Could you check a few things on this model? Use its own coordinates, in mm. A direction names the side the tool comes from. Round coordinates to 2 decimals unless told otherwise and drop trailing zeros. Loops run counter-clockwise (first coordinate to the right, second up) from the corner with the lowest first, then second, coordinate; pieces in that order, holes last. Notation, with made-up numbers: (59, 84) -> (66, 84) arc R18 cw to (66, 96) -> close; hole circle Ø11 at (-13, -22.5). An arc over 180 degrees is marked (long way). One line per item, written item: value.
```python
from build123d import *

# Parameters (mm, degrees)
F0_W      = 25
F0_H      = 90
F1_DEPTH  = 2
F2_R      = 2
F3_DEPTH  = 25
F4_W      = 25
F4_H      = 5
F5_DEPTH  = 2
F6_W      = 25
F6_H      = 2
F7_DEPTH  = 63
F8_R      = 5
F10_DEPTH = 25


with BuildPart() as f1:
    # F0 (on Front) → F1 (new body)
    with BuildSketch(Plane.XZ):
        Rectangle(F0_W, F0_H)
    extrude(amount=F1_DEPTH)

    # F2 (on face) → F3 (cut)
    with BuildSketch(Plane.XZ.offset(2)):
        with Locations((7.5, 25)):
            Circle(F2_R)
        with Locations((-6.5, -3)):
            Circle(F2_R)
    extrude(amount=-F3_DEPTH, mode=Mode.SUBTRACT)

    # F4 (on face) → F5 (join)
    with BuildSketch(Plane.XZ.offset(2)):
        with Locations((0, 47.5)):
            Rectangle(F4_W, F4_H)
    extrude(amount=-F5_DEPTH)

    # F6 (on face) → F7 (join)
    with BuildSketch(Plane.XZ.offset(2)):
        with Locations((0, 49)):
            Rectangle(F6_W, F6_H)
    extrude(amount=F7_DEPTH)

    # F8
    f8_edges = [f1.edges().sort_by_distance(p)[0] for p in [
        (-12.5, -65, 49),
        (12.5, -65, 49),
    ]]
    fillet(f8_edges, radius=F8_R)

    # F9 (on face) → F10 (cut)
    with BuildSketch(Plane.XY.offset(50)):
        with BuildLine():
            Line((-7.5, -49.8), (7.5, -49.8))
            ThreePointArc((7.5, -49.8), (10.5, -46.8), (7.5, -43.8))
            Line((7.5, -43.8), (-7.5, -43.8))
            ThreePointArc((-7.5, -43.8), (-10.5, -46.8), (-7.5, -49.8))
        make_face()
    extrude(amount=-F10_DEPTH, mode=Mode.SUBTRACT)


solid = f1.part
```
(1) We'd pull the mould along X, two halves only. Please class faces 1 (the face through (-11.07, -63.5, 49.01)), 2 (the face through (10.5, -46.9, 49)), 3 (the face through (0, 0, 3)): +X half, -X half, draft (parallel to the pull), parting line (faces both ways), or undercut.
Results below:
face 1: -X half
face 2: undercut
face 3: draft
(2) For pin 1 Ø2 at (x, y) = (-9.5, -9.5) entering from -Z; pin 2 Ø12.5 at (x, z) = (-4, 6.5) entering from -Y, each with a flat end and sliding along its axis, tell me the tip position at first contact or that it passes through.
Results below:
pin 1: stops at z = 48
pin 2: stops at y = -2
(3) Please list where these lines run through material, in increasing order: L1, parallel to Z at x = 8.5, y = -12; L2, parallel to Y at x = -1.5, z = -20; L3, parallel to Z at x = -6.5, y = -1.45.
Results below:
L1: z = 48 to 50
L2: y = -2 to 0
L3: z = -45 to -5, -1 to 50
(4) Imagine slicing it at C-C on x = -5.5. Write out the boundary of the cut face in (y, z).
Results below:
outline: (-65, 48) -> (-49.8, 48) -> (-49.8, 50) -> (-65, 50) -> close; (-43.8, 48) -> (-2, 48) -> (-2, -1.27) -> (0, -1.27) -> (0, 50) -> (-43.8, 50) -> close; (-2, -45) -> (0, -45) -> (0, -4.73) -> (-2, -4.73) -> close
(5) On a 3-axis mill with a long thin cutter (end or side, diameter ignored), from which of +Z, -Z, +X, -X, +Y, -Y can I reach the whole of each face in a straight line? I mean faces 4 (the face through (0, -2, 2)), 5 (the face through (-12.5, -1, 23)), 6 (the face through (0, -49.8, 49)). Say none if no direction works.
Results below:
face 4: -Z, +X, -X, -Y
face 5: +Z, -Z, -X, +Y, -Y
face 6: +Z, -Z
(6) Imagine slicing it at B-B on z = -3. Write out the boundary of the cut face in (x, y).
Results below:
outline: (-12.5, -2) -> (-8.5, -2) -> (-8.5, 0) -> (-12.5, 0) -> close; (-4.5, -2) -> (12.5, -2) -> (12.5, 0) -> (-4.5, 0) -> close
(7) Imagine slicing it at D-D on y = -8.5. Write out the boundary of the cut face in (x, z).
Results below:
outline: (-12.5, 48) -> (12.5, 48) -> (12.5, 50) -> (-12.5, 50) -> close
(8) Imagine slicing it at A-A on x = 1. Write out the boundary of the cut face in (y, z), then the cut area to 3 significant figures.
Results below:
outline: (-65, 48) -> (-49.8, 48) -> (-49.8, 50) -> (-65, 50) -> close; (-43.8, 48) -> (-2, 48) -> (-2, -45) -> (0, -45) -> (0, 50) -> (-43.8, 50) -> close
area: 304 mm²
